Source: CAD feature listing. Evaluate the final solid. Frame: model axes, mm. Face numbers are marked on the shaded views. A direction names the side the tool comes from. Give positions to 0.01 mm unless a question says otherwise; leave off trailing zeros. Loops run counter-clockwise (first coordinate to the right, second up) from the corner with the lowest first, then second, coordinate; pieces in that order, holes last.
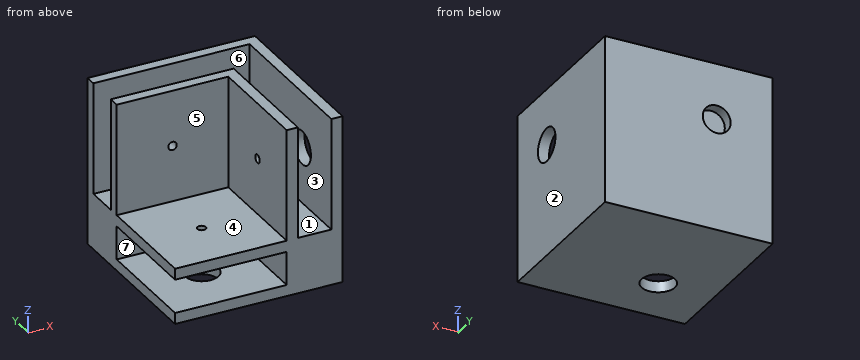
from build123d import *

# Parameters (mm, degrees)
F0_W      = 30
F0_H      = 30
F1_DEPTH  = 30
F2_W      = 20
F2_H      = 20
F3_DEPTH  = 20
F5_DEPTH  = 20
F6_W      = 20
F6_H      = 6
F7_DEPTH  = 20
F8_R      = 2.5
F9_DEPTH  = 2
F10_R     = 0.75
F11_DEPTH = 25
F12_R     = 3
F13_DEPTH = 2
F14_R     = 0.75
F15_DEPTH = 2
F16_R     = 0.75
F17_DEPTH = 2
F18_R     = 3
F19_DEPTH = 2


with BuildPart() as f1:
    # F0 (on Top) → F1 (new body)
    with BuildSketch(Plane.XY):
        with Locations((15, 15)):
            Rectangle(F0_W, F0_H)
    extrude(amount=F1_DEPTH)

    # F2 (on face) → F3 (cut)
    with BuildSketch(Plane.XY.offset(30)):
        with Locations((10, 10)):
            Rectangle(F2_W, F2_H)
    extrude(amount=-F3_DEPTH, mode=Mode.SUBTRACT)

    # F4 (on face) → F5 (cut)
    with BuildSketch(Plane.XY.offset(30)):
        Polygon((28, 28), (0, 28), (0, 22), (22, 22), (22, 0), (28, 0), (28, 22), align=None)
    extrude(amount=-F5_DEPTH, mode=Mode.SUBTRACT)

    # F6 (on face) → F7 (cut)
    with BuildSketch(Plane(origin=(0, 0, 0), x_dir=(0, -1, 0), z_dir=(-1, 0, 0))):
        with Locations((-10, 5)):
            Rectangle(F6_W, F6_H)
    extrude(amount=-F7_DEPTH, mode=Mode.SUBTRACT)

    # F8 (on face) → F9 (cut, through all)
    with BuildSketch(Plane(origin=(0, 30, 0), x_dir=(-1, 0, 0), z_dir=(0, 1, 0))):
        with Locations((-10, 20)):
            Circle(F8_R)
    extrude(amount=-F9_DEPTH, mode=Mode.SUBTRACT)

    # F10 (on face) → F11 (cut)
    with BuildSketch(Plane.XZ.offset(-20)):
        with Locations((10, 20)):
            Circle(F10_R)
    extrude(amount=-F11_DEPTH, mode=Mode.SUBTRACT)

    # F12 (on face) → F13 (cut, through all)
    with BuildSketch(Plane.YZ.offset(30)):
        with Locations((10, 20)):
            Circle(F12_R)
    extrude(amount=-F13_DEPTH, mode=Mode.SUBTRACT)

    # F14 (on face) → F15 (cut, through all)
    with BuildSketch(Plane(origin=(20, 0, 0), x_dir=(0, -1, 0), z_dir=(-1, 0, 0))):
        with Locations((-10, 20)):
            Circle(F14_R)
    extrude(amount=-F15_DEPTH, mode=Mode.SUBTRACT)

    # F16 (on face) → F17 (cut, through all)
    with BuildSketch(Plane.XY.offset(10)):
        with Locations((10, 10)):
            Circle(F16_R)
    extrude(amount=-F17_DEPTH, mode=Mode.SUBTRACT)

    # F18 (on face) → F19 (cut, through all)
    with BuildSketch(Plane(origin=(0, 0, 0), x_dir=(1, 0, 0), z_dir=(0, 0, -1))):
        with Locations((10, -10)):
            Circle(F18_R)
    extrude(amount=-F19_DEPTH, mode=Mode.SUBTRACT)


solid = f1.part
1) Ray query, probe 1 along X at (y, z) = (9.25, 16.25); probe 2 along Z at (x, y) = (29.35, 10); probe 3 along Y at (x, z) = (10, 1.35). Return the intervals inside material, ascending.
Checks:
probe 1: x = 20 to 22, 28 to 30
probe 2: z = 0 to 17, 23 to 30
probe 3: y = 0 to 7, 13 to 30
2) Pull-direction query (X, two-part tool) for the marked faces 1, 2, 3 and 4; classes: released by +X, released by -X, zero draft, split by the parting line, or undercut.
Checks:
face 1: undercut
face 2: released by +X
face 3: undercut
face 4: zero draft
3) Contact query for flat-ended pins moving along their axis: P1, Ø4.5, axis at x = 10, z = 20, coming from the -Y side; P2, Ø8, axis at x = 10, y = 10, coming from the -Z side; P3, Ø1.7, axis at x = 10, y = 10, coming from the +Z side; P4, Ø6, axis at y = 14, z = 24, coming from the -X side. Output: stop coordinate, or through.
Checks:
P1: stops at y = 20
P2: stops at z = 0
P3: stops at z = 10
P4: stops at x = 20
4) Reachability of the marked faces 5, 6 and 7 from +Z, -Z, +X, -X, +Y, -Y: full face, straight path, thin tool, end or side. Return the list, or none.
Checks:
face 5: +Z, -X, -Y
face 6: +Z, -X
face 7: -X, -Y
5) Cut plane B-B (y = 10). State how many separate pieces and enclosed holes the cut face has, and give its area (3 significant figures).
Checks:
separate pieces: 5
enclosed holes: 0
area: 230 mm2
6) Cut plane D-D (y = 21.25). Return loops of the section in (x, z), and give its area (3 significant figures).
Checks:
outline: (0, 0) - (30, 0) - (30, 30) - (28, 30) - (28, 10) - (22, 10) - (22, 30) - (0, 30) - close; hole circle Ø1.5 at (10, 20)
area: 778 mm2
7) Cut plane A-A (z = 20). Return loops of the section in (x, y).
Checks:
outline: (0, 20) - (9.25, 20) - (9.25, 22) - (0, 22) - close; (0, 28) - (7.5, 28) - (7.5, 30) - (0, 30) - close; (10.75, 20) - (20, 20) - (20, 10.75) - (22, 10.75) - (22, 22) - (10.75, 22) - close; (12.5, 28) - (28, 28) - (28, 13) - (30, 13) - (30, 30) - (12.5, 30) - close; (20, 0) - (22, 0) - (22, 9.25) - (20, 9.25) - close; (28, 0) - (30, 0) - (30, 7) - (28, 7) - close
